```python
from build123d import *

# Parameters (mm, degrees)
SKETCH1_R           = 4
BOSS_EXTRUDE1_DEPTH = 30
SKETCH2_R           = 7
BOSS_EXTRUDE2_DEPTH = 5.5
BOSS_EXTRUDE2_TAPER = 30
CUT_EXTRUDE1_DEPTH  = 3.8
SKETCH4_R           = 2.65
CUT_EXTRUDE2_DEPTH  = 22
CHAMFER1_SIZE       = 0.3
FILLET1_R           = 0.3


with BuildPart() as part:
    # Sketch1 → Boss-Extrude1 (new body)
    with BuildSketch(Plane(origin=(0, 0, 0), x_dir=(1, 0, 0), z_dir=(0, 1, 0))):
        with Locations(Location((0, 0, 0), (0, 0, 270))):
            Circle(SKETCH1_R)
    extrude(amount=BOSS_EXTRUDE1_DEPTH)

    # Sketch2 → Boss-Extrude2 (add)
    with BuildSketch(Plane(origin=(0, 30, 0), x_dir=(1, 0, 0), z_dir=(0, 1, 0))):
        Circle(SKETCH2_R)
    extrude(amount=BOSS_EXTRUDE2_DEPTH, taper=BOSS_EXTRUDE2_TAPER)

    # Sketch3 → Cut-Extrude1 (cut)
    with BuildSketch(Plane(origin=(0, 35.5, 0), x_dir=(1, 0, 0), z_dir=(0, 1, 0))):
        Polygon((0, 3.0022214), (-2.6, 1.5011107), (-2.6, -1.5011107), (0, -3.0022214), (2.6, -1.5011107), (2.6, 1.5011107), align=None)
    extrude(amount=-CUT_EXTRUDE1_DEPTH, mode=Mode.SUBTRACT)

    # Sketch4 → Cut-Extrude2 (cut)
    with BuildSketch(Plane.XZ):
        with Locations(Location((0, 0, 0), (0, 0, 270))):
            Circle(SKETCH4_R)
    extrude(amount=-CUT_EXTRUDE2_DEPTH, mode=Mode.SUBTRACT)

    # Chamfer1
    chamfer1_edges = [part.edges().sort_by_distance(p)[0] for p in [
        (0, 0, -4),
    ]]
    chamfer(chamfer1_edges, length=CHAMFER1_SIZE)

    # Fillet1
    fillet1_edges = [part.edges().sort_by_distance(p)[0] for p in [
        (-7, 30, 0),
    ]]
    fillet(fillet1_edges, radius=FILLET1_R)


solid = part.part
```
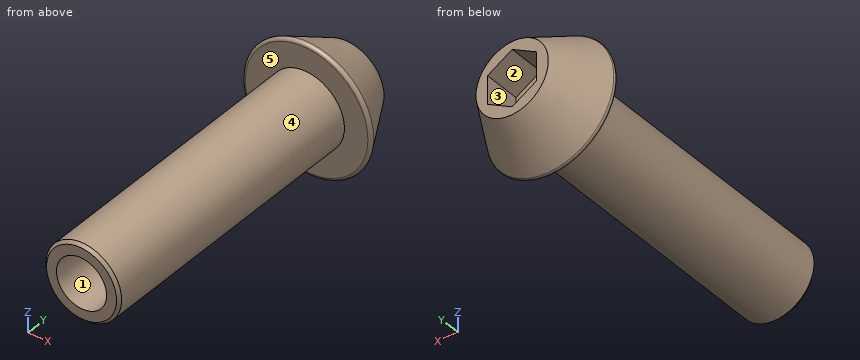
Model file for the job. Use its own axes, mm. Face numbers are marked on the shaded views. A direction names the side the tool comes from. Give positions to 0.01 mm unless a question says otherwise; leave off trailing zeros. Loops run counter-clockwise (first coordinate to the right, second up) from the corner with the lowest first, then second, coordinate; pieces in that order, holes last. Notation, with made-up numbers: M 62.5,-14 L 78.5,-14 A24 ccw 78.5,6 Z; hole C 32.5,-30 d2. An arc over 180 degrees is marked long. Use one line per item in the form item = value.
Item 1: Slice it at A-A on y = 5.5. List the corners of the cut face in (x, z), and give its area (3 significant figures).
Filled in:
outline = C 0,0 d8; hole C 0,0 d5.3
area = 28.2 mm^2
Item 2: Slice it at B-B on y = 27.5. List the corners of the cut face in (x, z).
Filled in:
outline = C 0,0 d8
Item 3: Drill centre lines: L1, parallel to X at y = 6, z = 0; L2, parallel to Y at x = -2.5, z = 1; L3, parallel to Y at x = -1.25, z = -1. Where is each one in solid material? Low to high.
Filled in:
L1 = -4 to -2.65, 2.65 to 4
L2 = 0 to 31.7
L3 = 22 to 31.7
Item 4: Flat gauge pins, fed straight in: pin 1 Ø4 at (x, z) = (0, 0) entering from -Y; pin 2 Ø2 at (y, z) = (20.5, -4) entering from +X; pin 3 Ø3.5 at (y, z) = (34, 0) entering from +X. Where does each tip first touch, or does it go through?
Filled in:
pin_1 = 22
pin_2 = 2.65
pin_3 = 5.7
Item 5: Which spindle directions (+Z, -Z, +X, -X, +Y, -Y) get a long thin tool onto all of the face, cutting with end or side? Do the marked faces 1 and 2. Say none if no direction does.
Filled in:
face_1 = -Y
face_2 = +Y
Item 6: Two-plate mould, pull along X, no slides. Class the marked faces 3, 4 and 5: released by +X, released by -X, zero draft, split by the parting line, or undercut.
Filled in:
face_3 = undercut
face_4 = split by the parting line
face_5 = zero draft
